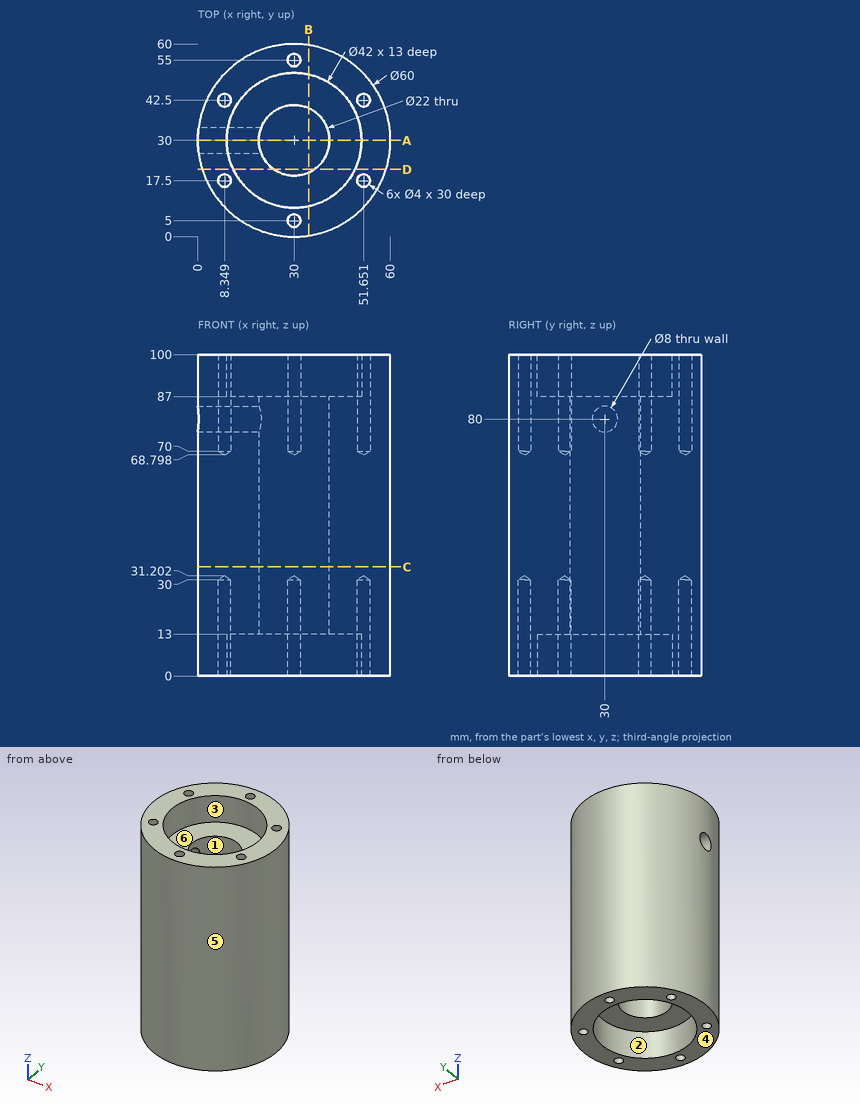
Design review of the part shown in the three views and the two pictorial views. Dimensions are in mm from the part's minimum x, y and z. A direction names the side the tool comes from. Round coordinates to 2 decimals unless told otherwise and drop trailing zeros. Write each loop counter-clockwise with the first axis right and the second up, starting at its lowest first coordinate (ties: lowest second). Pieces come first, ordered by that corner, then holes. Notation, with made-up numbers: (61.25, 59.5) -> (93.25, 59.5) arc R5 ccw to (93.25, 65.5) -> close; hole circle Ø2 at (-19.5, 41). An arc over 180 degrees is marked (long way). One line per question, with ' | ' between items. Start each with the question number.
1) Add section D-D (y = 21). Write out the cut boundary in (x, z) (1 decimal).
2) For pin 1 Ø6 at (x, z) = (53, 55) entering from -Y; pin 2 Ø3 at (y, z) = (10.5, 34) entering from +X; pin 3 Ø6.5 at (x, y) = (30, 55) entering from +Z; pin 4 Ø3 at (x, y) = (51.65, 42.5) entering from -Z, all flat-tipped, find the tip position at first contact; note any pin that passes through.
3) Wall thickness on line 1 along Y through (x, z) = (30, 76); line 2 along Y through (x, z) = (30, 10.5); line 3 along Y through (x, z) = (30, 51): over which ranges is each line inside the solid? List them lowest first.
4) Add section A-A (y = 30). Write out the cut boundary in (x, z).
5) Add section C-C (z = 34). Write out the cut boundary in (x, y), and give its area (3 significant figures).
6) Mouldability with a two-part tool opening along Y and no side actions: class the marked faces 4, 5 and 6 as +Y half, -Y half, draft (parallel to the pull), parting line (faces both ways), or undercut.
7) Add section B-B (x = 34.5). Write out the cut boundary in (y, z).
8) Machinability: for the marked faces 1, 2 and 3, which of the approach directions +Z, -Z, +X, -X, +Y, -Y give a long, thin tool a straight path to every point of the face, cutting with its end or side? Answer none if there is none.
Reported:
1) outline: (1.4, 0) -> (11, 0) -> (11, 13) -> (23.7, 13) -> (23.7, 87) -> (11, 87) -> (11, 100) -> (1.4, 100) -> close; (36.3, 13) -> (49, 13) -> (49, 0) -> (58.6, 0) -> (58.6, 100) -> (49, 100) -> (49, 87) -> (36.3, 87) -> close
2) pin 1: stops at y = 7.64 | pin 2: stops at x = 54 | pin 3: stops at z = 100 | pin 4: stops at z = 30.3
3) line 1: y = 0 to 3, 7 to 19, 41 to 53, 57 to 60 | line 2: y = 0 to 3, 7 to 9, 51 to 53, 57 to 60 | line 3: y = 0 to 19, 41 to 60
4) outline: (0, 0) -> (9, 0) -> (9, 13) -> (19, 13) -> (19, 76) -> (0, 76) -> close; (0, 84) -> (19, 84) -> (19, 87) -> (9, 87) -> (9, 100) -> (0, 100) -> close; (41, 13) -> (51, 13) -> (51, 0) -> (60, 0) -> (60, 100) -> (51, 100) -> (51, 87) -> (41, 87) -> close
5) outline: circle Ø60 at (30, 30); hole circle Ø22 at (30, 30) | area: 2,450 mm²
6) face 4: draft | face 5: parting line | face 6: undercut
7) outline: (0.34, 0) -> (9.49, 0) -> (9.49, 13) -> (19.96, 13) -> (19.96, 87) -> (9.49, 87) -> (9.49, 100) -> (0.34, 100) -> close; (40.04, 13) -> (50.51, 13) -> (50.51, 0) -> (59.66, 0) -> (59.66, 100) -> (50.51, 100) -> (50.51, 87) -> (40.04, 87) -> close
8) face 1: +Z, -Z | face 2: -Z | face 3: +Z
